from build123d import *

# Parameters (mm, degrees)
SKETCH2_R          = 5
CUT_EXTRUDE1_DEPTH = 110.819169547


with BuildPart() as part:
    # Sketch1 → Revolve1 (revolve)
    with BuildSketch(Plane(origin=(0, 0, 0), x_dir=(0, 0, -1), z_dir=(1, 0, 0)), mode=Mode.PRIVATE) as revolve1_sk:
        Polygon((0, 25), (0, 20), (24, 20), (24, 15), (33.5, 15), (33.5, 17), (35.5, 17), (35.5, 15), (48, 15), (48, 18.5), (51.5, 18.5), (51.5, 15), (63.5, 15), (63.5, 17), (65.5, 17), (65.5, 15), (86, 15), (89.5, 18.5), (89.5, 23), (83.5, 23), (83.5, 27), (89.5, 27), (89.5, 45), (75.5, 45), (75.5, 20), (31.5, 20), (31.5, 25), align=None)
    revolve(revolve1_sk.sketch.rotate(Axis((0, 0, -114.136596419), (0, 0, 1)), 90), axis=Axis((0, 0, -114.136596419), (0, 0, 1)))

    # Sketch2 → Cut-Extrude1 (cut, through all)
    with BuildSketch(Plane(origin=(0, 0, -89.5), x_dir=(-1, 0, 0), z_dir=(0, 0, -1))):
        with Locations((0, 35)):
            Circle(SKETCH2_R)
        with Locations((35, 0)):
            Circle(SKETCH2_R)
        with Locations((0, -35)):
            Circle(SKETCH2_R)
        with Locations((-35, 0)):
            Circle(SKETCH2_R)
    extrude(amount=-CUT_EXTRUDE1_DEPTH, mode=Mode.SUBTRACT)


solid = part.part
Geometry check sheet. Reference: the model listing, model coordinates, mm. A direction names the side the tool comes from. Round coordinates to 2 decimals unless told otherwise and drop trailing zeros. Loops run counter-clockwise (first coordinate to the right, second up) from the corner with the lowest first, then second, coordinate; pieces in that order, holes last.
Item 1: Cross-section at A-A on y = 37. Record the boundary of the cut face in (x, z), then the cut area to 3 significant figures.
Item 2: Cross-section at B-B on x = 35. Record the boundary of the cut face in (y, z), then the cut area to 3 significant figures.
Item 3: Access from +Z, -Z, +X, -X, +Y, -Y to the whole of each face (thin tool, end or side, straight path). Record for faces 5 (the flat face through (-3, -15, -24)), 6 (the flat face through (6, 14, -33.5)), 7 (the flat face through (19.4, 19.4, -89.5)).
Item 4: Mould release check, pull along Z, two halves, no side actions. Record for faces 1 (the cylindrical face through (-20.765, 39.923, -82.402)), 2 (the flat face through (-6, 14, -35.5)), 3 (the flat face through (6, 14, -63.5)), 4 (the flat face through (20, -12, -83.5)): pulls with the +Z half, pulls with the -Z half, needs draft (parallel to the pull), parting line crosses it, or undercut.
Item 5: Gauge pin test, flat ends, axial feed: pin 1 (18 mm diameter, centred on x = 0, y = 0, fed in from -Z); pin 2 (3 mm diameter, centred on y = -13.5, z = -25.5, fed in from -X); pin 3 (12 mm diameter, centred on y = 25.5, z = -9, fed in from -X); pin 4 (17 mm diameter, centred on x = 8.5, y = -1, fed in from -Z). Record the tip position at first contact, or that the pin passes through.
Item 6: Cross-section at C-C on z = -30. Record the boundary of the cut face in (x, y), then the cut area to 3 significant figures.
Item 7: Cross-section at D-D on x = 0. Count the separate pieces of the cut face and the enclosed holes in it, then the cut area to 3 significant figures.
Item 8: Thickness scan on line 1 (Y direction, x = 0, z = -5); line 2 (Y direction, x = 0, z = -34); line 3 (Z direction, x = -19, y = 11). Record the ranges inside material, lowest first.
Answer sheet:
1. outline: (-25.61, -89.5) - (-4.58, -89.5) - (-4.58, -75.5) - (-25.61, -75.5) - close; (4.58, -89.5) - (25.61, -89.5) - (25.61, -75.5) - (4.58, -75.5) - close
1. area: 589 mm2
2. outline: (-28.28, -89.5) - (-5, -89.5) - (-5, -75.5) - (-28.28, -75.5) - close; (5, -89.5) - (28.28, -89.5) - (28.28, -75.5) - (5, -75.5) - close
2. area: 652 mm2
3. face 5: +Z
3. face 6: none
3. face 7: -Z, +X, -X, +Y, -Y
4. face 1: needs draft
4. face 2: undercut
4. face 3: undercut
4. face 4: pulls with the -Z half
5. pin 1: passes through
5. pin 2: stops at x = -21.93
5. pin 3: stops at x = -15.64
5. pin 4: stops at z = -88.06
6. outline: circle Ø50 at (0, 0); hole circle Ø30 at (0, 0)
6. area: 1,260 mm2
7. separate pieces: 4
7. enclosed holes: 0
7. area: 1,290 mm2
8. line 1: y = -25 to -20, 20 to 25
8. line 2: y = -20 to -17, 17 to 20
8. line 3: z = -89.5 to -75.5, -31.5 to 0
